Geometry check sheet. Reference: drawing and pictorial views, mm from the part's lowest x, y, z. A direction names the side the tool comes from. Give positions to 0.01 mm unless a question says otherwise; leave off trailing zeros. Loops run counter-clockwise (first coordinate to the right, second up) from the corner with the lowest first, then second, coordinate; pieces in that order, holes last. Notation, with made-up numbers: (75.25, -35) - (96.25, -35) arc R28 ccw to (96.25, 4) - close; hole circle Ø3 at (83, -39). An arc over 180 degrees is marked (long way). Answer in a Markdown table with one row per item. Add a question column.
(1) Thickness scan on L1, parallel to Z at x = 10, y = 1.8 (3 decimals); L2, parallel to Z at x = 10, y = 0.3; L3, parallel to X at y = 1.5, z = 10. Record the ranges inside material, lowest first.
(2) Go/stop test with flat-tipped pins: P1, Ø4, axis at x = 10, z = 16, coming from the +Y side; P2, Ø2.5, axis at x = 10, z = 4, coming from the +Y side. Record where each tip stops, or that it passes through.
(3) Sectioned sample at C-C on y = 0.75. Enter the section's corners in (x, z), then the cut area to 3 significant figures.
(4) Sectioned sample at A-A on z = 4. Enter the section's corners in (x, y) (3 decimals).
(5) Set-up check for the marked faces 1 and 2: record each of +Z, -Z, +X, -X, +Y, -Y from which the full face is reachable in a straight line by a thin tool's end or side.
(6) Sectioned sample at B-B on x = 10. Enter the section's corners in (y, z) (3 decimals).
(7) Draft check along Z on the marked faces 3, 4 and 5. Enter one of: released by +Z, released by -Z, zero draft, split by the parting line, or undercut.
(8) Sectioned sample at D-D on z = 15.75. Enter the section's corners in (x, y), then the cut area to 3 significant figures.
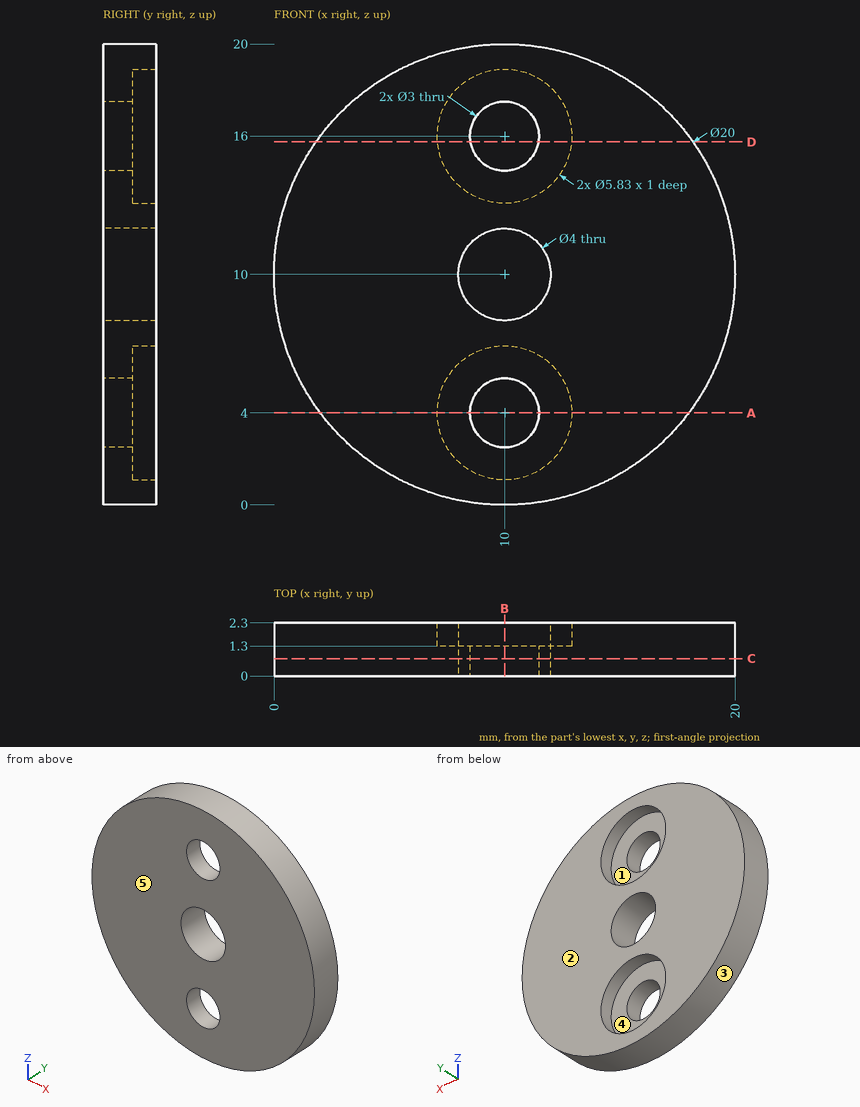
Reply:
| question | item | result |
|---|---|---|
| 1 | L1 | 0 to 1.085, 6.915 to 8, 12 to 13.085, 18.915 to 20 |
| 1 | L2 | 0 to 2.5, 5.5 to 8, 12 to 14.5, 17.5 to 20 |
| 1 | L3 | 0 to 8, 12 to 20 |
| 2 | P1 | y = 1.3 |
| 2 | P2 | through |
| 3 | outline | circle Ø20 at (10, 10); hole circle Ø4 at (10, 10); hole circle Ø3 at (10, 4); hole circle Ø3 at (10, 16) |
| 3 | area | 287 mm^2 |
| 4 | outline | (2, 0) - (8.5, 0) - (8.5, 1.3) - (7.085, 1.3) - (7.085, 2.3) - (2, 2.3) - close; (11.5, 0) - (18, 0) - (18, 2.3) - (12.915, 2.3) - (12.915, 1.3) - (11.5, 1.3) - close |
| 5 | face 1 | +Y |
| 5 | face 2 | +Z, -Z, +X, -X, +Y |
| 6 | outline | (0, 0) - (2.3, 0) - (2.3, 1.085) - (1.3, 1.085) - (1.3, 2.5) - (0, 2.5) - close; (0, 5.5) - (1.3, 5.5) - (1.3, 6.915) - (2.3, 6.915) - (2.3, 8) - (0, 8) - close; (0, 12) - (2.3, 12) - (2.3, 13.085) - (1.3, 13.085) - (1.3, 14.5) - (0, 14.5) - close; (0, 17.5) - (1.3, 17.5) - (1.3, 18.915) - (2.3, 18.915) - (2.3, 20) - (0, 20) - close |
| 7 | face 3 | split by the parting line |
| 7 | face 4 | undercut |
| 7 | face 5 | zero draft |
| 8 | outline | (1.82, 0) - (8.52, 0) - (8.52, 1.3) - (7.1, 1.3) - (7.1, 2.3) - (1.82, 2.3) - close; (11.48, 0) - (18.18, 0) - (18.18, 2.3) - (12.9, 2.3) - (12.9, 1.3) - (11.48, 1.3) - close |
| 8 | area | 28.0 mm^2 |
